from build123d import *

# Parameters (mm, degrees)
F0_W     = 457.2
F0_H     = 203.2
F1_DEPTH = 12.7
F2_R     = 6.35
F3_DEPTH = 25.4


with BuildPart() as f1:
    # F0 (on Top) → F1 (new body)
    with BuildSketch(Plane.XY):
        Rectangle(F0_W, F0_H)
    extrude(amount=-F1_DEPTH)

    # F2 (on face) → F3 (cut)
    with BuildSketch(Plane.XY):
        Circle(F2_R)
        with Locations((0, 50.8)):
            Circle(F2_R)
        with Locations((101.59225, -1.254837)):
            Circle(F2_R)
        with Locations((101.59225, 49.545163)):
            Circle(F2_R)
        with Locations((203.1845, -2.509675)):
            Circle(F2_R)
        with Locations((203.1845, 48.290325)):
            Circle(F2_R)
        with Locations((101.59225, -49.545163)):
            Circle(F2_R)
        with Locations((203.1845, -48.290325)):
            Circle(F2_R)
        with Locations((0, -50.8)):
            Circle(F2_R)
        with Locations((-101.59225, -1.254837)):
            Circle(F2_R)
        with Locations((-101.59225, -49.545163)):
            Circle(F2_R)
        with Locations((-203.1845, -48.290325)):
            Circle(F2_R)
        with Locations((-101.59225, 49.545163)):
            Circle(F2_R)
        with Locations((-203.1845, -2.509675)):
            Circle(F2_R)
        with Locations((-203.1845, 48.290325)):
            Circle(F2_R)
    extrude(amount=-F3_DEPTH, mode=Mode.SUBTRACT)


solid = f1.part
The listing builds one solid part. Answer for the finished solid, in the listing's coordinates (mm). Round coordinates to 2 decimals unless told otherwise and drop trailing zeros. Order: outer loops, then holes, each group sorted by start corner. A loop starts at its lowest first (then second) coordinate and runs counter-clockwise, first axis right, second up. Notation, with made-up numbers: M 79,46 L 93,46 A29 ccw 93,85 Z; hole C 50,41 d2. An arc over 180 degrees is marked long. Answer in a Markdown table with one row per item. Add a question column.
1) Determine the mould class of faces 1 (the face through (-3, -101.6, -6)), 2 (the face through (95.25, -0.98, -6.26)), 3 (the face through (-3, 101.6, -6)) for opening direction Y: pulls with the +Y half, pulls with the -Y half, needs draft (parallel to the pull), parting line crosses it, or undercut.
2) Consider line 1 along Y through (x, z) = (207.5, -3.75); line 2 along Y through (x, z) = (200, -2.5); line 3 along X through (y, z) = (-53.5, -7.5). Determine where each line is inside the solid, lowest interval first. Write a range as from..to.
3) The part is cut by section B-B on z = -8.75. Count the separate pieces of the cut face and the enclosed holes in it, plus the area to 3 significant figures.
4) A flat-ended cylindrical pin translates along its axis: pin 1 Ø16.5 at (x, y) = (203.18, 48.29) entering from -Z. Find the tip coordinate at first contact, or state that the pin passes through.
5) The part is cut by section A-A on x = 0. Determine the outline of the cut face in (y, z), plus the area to 3 significant figures.
Findings below:
| question | item | result |
|---|---|---|
| 1 | face 1 | pulls with the -Y half |
| 1 | face 2 | undercut |
| 1 | face 3 | pulls with the +Y half |
| 2 | line 1 | y = -101.6..-52.95, -43.63..-7.17, 2.15..43.63, 52.95..101.6 |
| 2 | line 2 | y = -101.6..-53.78, -42.8..-8, 2.98..42.8, 53.78..101.6 |
| 2 | line 3 | x = -228.6..-206.82, -199.55..-106.56, -96.62..-5.75, 5.75..96.62, 106.56..199.55, 206.82..228.6 |
| 3 | separate pieces | 1 |
| 3 | enclosed holes | 15 |
| 3 | area | 91,000 mm² |
| 4 | pin 1 | stops at z = -12.7 |
| 5 | outline | M -101.6,-12.7 L -57.15,-12.7 L -57.15,0 L -101.6,0 Z; M -44.45,-12.7 L -6.35,-12.7 L -6.35,0 L -44.45,0 Z; M 6.35,-12.7 L 44.45,-12.7 L 44.45,0 L 6.35,0 Z; M 57.15,-12.7 L 101.6,-12.7 L 101.6,0 L 57.15,0 Z |
| 5 | area | 2,100 mm² |
